The figure shows three views and two pictorial views of one solid part (mm, origin at its lowest corner). Answer the questions. Give positions to 0.01 mm unless a question says otherwise; leave off trailing zeros. Write each loop counter-clockwise with the first axis right and the second up, starting at its lowest first coordinate (ties: lowest second). Pieces come first, ordered by that corner, then holes. Notation, with made-up numbers: (46, 21) - (72, 21) arc R10 ccw to (72, 31) - close; hole circle Ø1 at (10, 47). An arc over 180 degrees is marked (long way). One line per question, with ' | ' between items. Start each with the question number.
1. A cutting plane is placed at B-B (x = 17). Determine the outline of the cut face in (y, z).
2. A cutting plane is placed at A-A (y = 17). State how many separate pieces and enclosed holes the cut face has, then the cut area to 3 significant figures.
3. Given P1, Ø2.5, axis at y = 17, z = 35, coming from the -X side; P2, Ø3, axis at x = 12, z = 6.5, coming from the +Y side; P3, Ø8, axis at x = 25.5, z = 22, coming from the -Y side, each flat-ended and moving along its own axis, determine where each tip first touches the part or whether it passes through.
4. Find the intervals of material crossed by L1, parallel to X at y = 17.5, z = 27.5; L2, parallel to Z at x = 17, y = 32.2; L3, parallel to Z at x = 31, y = 8.5, in increasing order. Write a range as from..to.
5. A cutting plane is placed at C-C (z = 35). Determine the outline of the cut face in (x, y), then the cut area to 3 significant figures.
6. A cutting plane is placed at D-D (x = 22). Determine the outline of the cut face in (y, z), then the cut area to 3 significant figures.
7. The mould has two halves that part along Y. Classify the marked faces 1, 2 and 3: +Y half, -Y half, draft (parallel to the pull), parting line (faces both ways), or undercut.
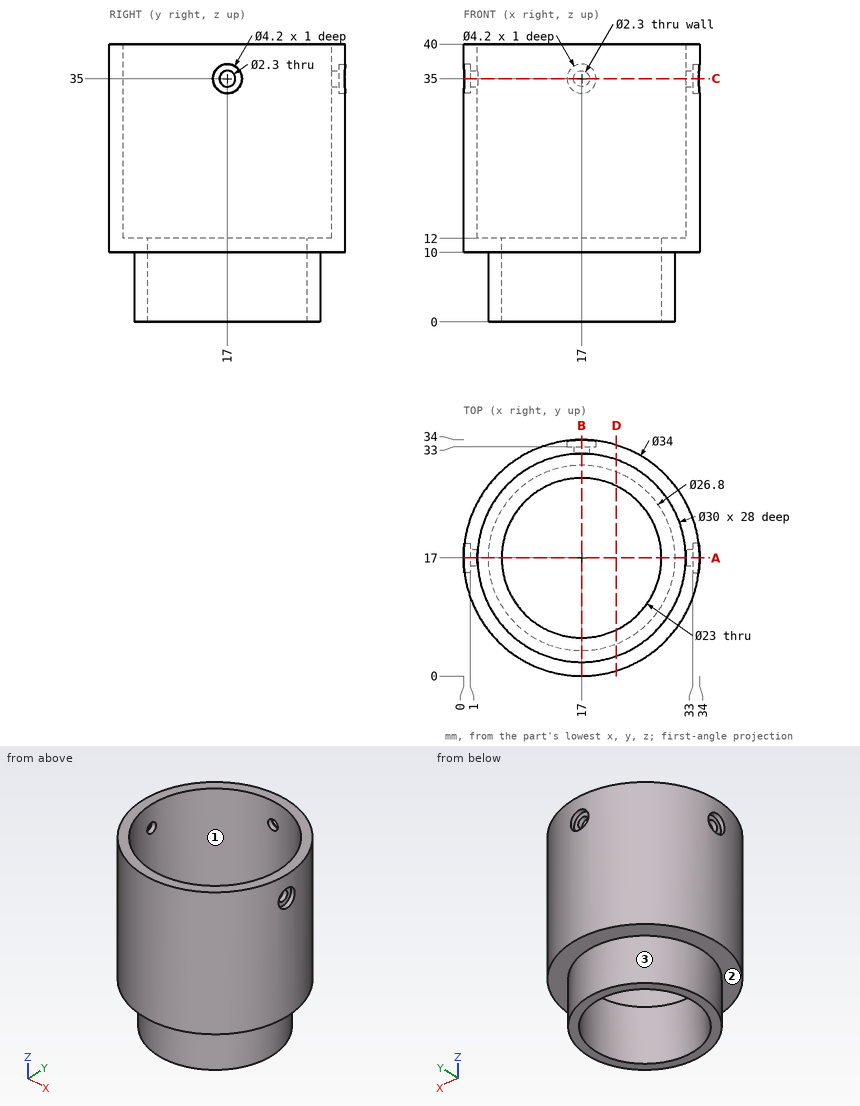
Determined:
1) outline: (0, 10) - (3.6, 10) - (3.6, 0) - (5.5, 0) - (5.5, 12) - (2, 12) - (2, 40) - (0, 40) - close; (28.5, 0) - (30.4, 0) - (30.4, 10) - (34, 10) - (34, 32.9) - (33, 32.9) - (33, 33.85) - (32, 33.85) - (32, 12) - (28.5, 12) - close; (32, 36.15) - (33, 36.15) - (33, 37.1) - (34, 37.1) - (34, 40) - (32, 40) - close
2) separate pieces: 4 | enclosed holes: 0 | area: 159 mm2
3) P1: x = 1 | P2: y = 29.93 | P3: y = 0.61
4) L1: 0.01..2.01, 31.99..33.99 | L2: 10..33.85, 36.15..40 | L3: 10..40
5) outline: (0.13, 14.9) arc R17 ccw to (33.87, 14.9) - (33, 14.9) - (33, 15.85) - (31.96, 15.85) arc R15 cw to (2.04, 15.85) - (1, 15.85) - (1, 14.9) - close; (0.13, 19.1) - (1, 19.1) - (1, 18.15) - (2.04, 18.15) arc R15 cw to (15.85, 31.96) - (15.85, 33) - (14.9, 33) - (14.9, 33.87) arc R17 ccw to start; (18.15, 31.96) arc R15 cw to (31.96, 18.15) - (33, 18.15) - (33, 19.1) - (33.87, 19.1) arc R17 ccw to (19.1, 33.87) - (19.1, 33) - (18.15, 33) - close | area: 182 mm2
6) outline: (0.75, 10) - (4.57, 10) - (4.57, 0) - (6.64, 0) - (6.64, 12) - (2.86, 12) - (2.86, 40) - (0.75, 40) - close; (27.36, 0) - (29.43, 0) - (29.43, 10) - (33.25, 10) - (33.25, 40) - (31.14, 40) - (31.14, 12) - (27.36, 12) - close | area: 183 mm2
7) face 1: undercut | face 2: draft | face 3: parting line
